Geometry check sheet. Reference: drawing and pictorial views, mm from the part's lowest x, y, z. A direction names the side the tool comes from. Give positions to 0.01 mm unless a question says otherwise; leave off trailing zeros. Order: outer loops, then holes, each group sorted by start corner. A loop starts at its lowest first (then second) coordinate and runs counter-clockwise, first axis right, second up.
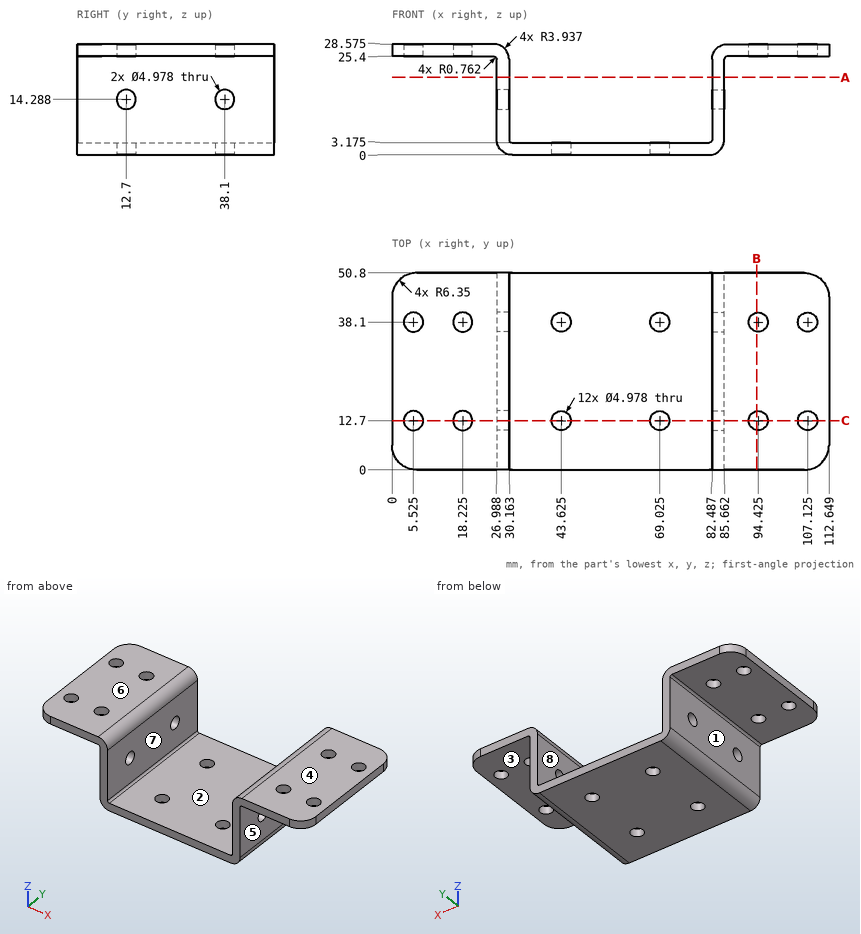
(1) Set-up check for the marked faces 1, 2, 3 and 4: record each of +Z, -Z, +X, -X, +Y, -Y from which the full face is reachable in a straight line by a thin tool's end or side.
Response values:
face 1: -Z, -X, +Y, -Y
face 2: +Z, +Y, -Y
face 3: -Z, +X, +Y, -Y
face 4: +Z, +X, -X, +Y, -Y
(2) Cross-section at C-C on y = 12.7. Count the separate pieces of the cut face and the enclosed holes in it.
Response values:
separate pieces: 9
enclosed holes: 0
(3) Release check for a two-part mould opening along X. For the marked faces 5, 6, 7 and 8 record: released by +X, released by -X, zero draft, split by the parting line, or undercut.
Response values:
face 5: released by +X
face 6: zero draft
face 7: undercut
face 8: undercut
(4) Material ranges on L1, parallel to X at y = 9.5, z = 19.75; L2, parallel to X at y = 37.5, z = 3; L3, parallel to Z at x = 88.5, y = 40.5 (1 decimal), recorded low to high.
Response values:
L1: x = 26.99 to 30.16, 82.49 to 85.66
L2: x = 27.1 to 41.21, 46.04 to 66.61, 71.44 to 85.55
L3: z = 25.4 to 28.6
(5) Cross-section at A-A on z = 20. Enter the section's corners in (x, y).
Response values:
outline: (26.99, 0) - (30.16, 0) - (30.16, 50.8) - (26.99, 50.8) - close; (82.49, 0) - (85.66, 0) - (85.66, 50.8) - (82.49, 50.8) - close
(6) Cross-section at B-B on x = 94. Enter the section's corners in (y, z) (1 decimal), then the cut area to 3 significant figures.
Response values:
outline: (0, 25.4) - (10.2, 25.4) - (10.2, 28.6) - (0, 28.6) - close; (15.2, 25.4) - (35.6, 25.4) - (35.6, 28.6) - (15.2, 28.6) - close; (40.6, 25.4) - (50.8, 25.4) - (50.8, 28.6) - (40.6, 28.6) - close
area: 130 mm2
(7) Gauge pin test, flat ends, axial feed: pin 1 Ø15 at (x, y) = (52.5, 16.5) entering from +Z (1 decimal); pin 2 Ø5.5 at (y, z) = (38.1, 14.29) entering from -X; pin 3 Ø13 at (x, y) = (99, 14.5) entering from -Z. Record the tip position at first contact, or that the pin passes through.
Response values:
pin 1: stops at z = 3.2
pin 2: stops at x = 26.99
pin 3: stops at z = 25.4
